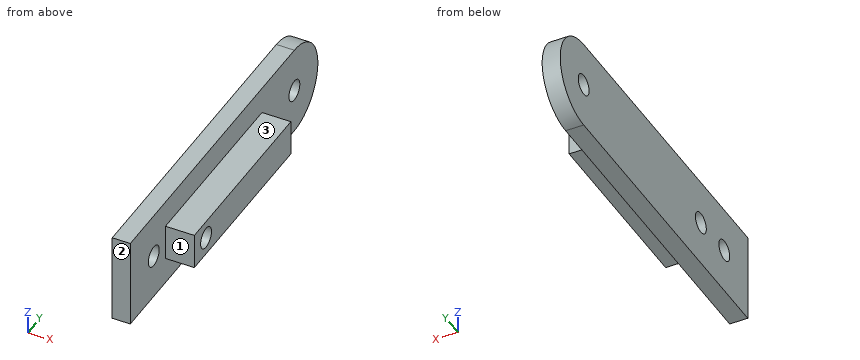
```python
from build123d import *

# Parameters (mm, degrees)
BOSS_EXTRUDE1_DEPTH     = 2.54
SKETCH2_W               = 5.08
SKETCH2_H               = 26.152706233
BOSS_EXTRUDE2_DEPTH     = 4.064
CUT_EXTRUDE1_DEPTH      = 46.384334478
CUT_EXTRUDE1_DEPTH_BACK = 46.384334478
SKETCH3_R               = 1.4732
F_4_CLEARANCE_HOLE1_D   = 2.9464


with BuildPart() as part:
    # Sketch1 → Boss-Extrude1 (new body)
    with BuildSketch(Plane(origin=(0, 0, 0), x_dir=(0, 0, -1), z_dir=(1, 0, 0))):
        with BuildLine():
            Line((-6.35, 0), (-6.35, -44.45))
            Line((-6.35, -44.45), (6.35, -44.45))
            Line((6.35, -44.45), (6.35, 0))
            ThreePointArc((6.35, 0), (0, 6.35), (-6.35, 0))
        make_face()
    extrude(amount=BOSS_EXTRUDE1_DEPTH)

    # Sketch2 → Boss-Extrude2 (add)
    with BuildSketch(Plane(origin=(2.54, 0, 0), x_dir=(0, 0, -1), z_dir=(1, 0, 0))):
        with Locations((0, -21.848646884)):
            Rectangle(SKETCH2_W, SKETCH2_H)
    extrude(amount=BOSS_EXTRUDE2_DEPTH)

    # Sketch3 → Cut-Extrude1 (cut, two sides: drawn at the far end of the back side and taken through both)
    with BuildSketch(Plane.ZY.offset(-CUT_EXTRUDE1_DEPTH_BACK)):
        Circle(SKETCH3_R)
    extrude(amount=CUT_EXTRUDE1_DEPTH + CUT_EXTRUDE1_DEPTH_BACK, mode=Mode.SUBTRACT)

    # #4 Clearance Hole1 (through all)
    with Locations(Plane.ZY):
        with Locations((0, -31.75), (0, -38.1)):
            Hole(F_4_CLEARANCE_HOLE1_D / 2)


solid = part.part
```
Can you work these out from the model? Positions are in its coordinate system, mm. Face numbers are marked on the shaded views. A direction names the side the tool comes from. Round coordinates to 2 decimals unless told otherwise and drop trailing zeros. Loops run counter-clockwise (first coordinate to the right, second up) from the corner with the lowest first, then second, coordinate; pieces in that order, holes last. Notation, with made-up numbers: M 16,42 L 71,42 A29 cw 71,67 Z; hole C -15.75,-34 d1. An arc over 180 degrees is marked long. Answer as a JSON object with one key per item and string values. Group by question number.
Q1. On a 3-axis mill with a long thin cutter (end or side, diameter ignored), from which of +Z, -Z, +X, -X, +Y, -Y can I reach the whole of each face in a straight line? I mean the marked faces 1, 2 and 3. Say none if no direction works.
Q2. Please list where these lines run through material, in increasing order: L1, parallel to Y at x = 0.75, z = 0; L2, parallel to Y at x = 3, z = 0 (3 decimals); L3, parallel to X at y = 2, z = -5.5.
Q3. Will these pins go through, and if not, where does the flat tip stop? pin 1 (2 mm diameter, centred on x = 4, y = -26, fed in from +Z); pin 2 (2.5 mm diameter, centred on y = -38.1, z = 0, fed in from -X); pin 3 (1 mm diameter, centred on x = 4, z = -2, fed in from -Y) (3 decimals); pin 4 (3 mm diameter, centred on y = -38, z = 4, fed in from +X).
Q4. Imagine slicing it at A-A, the plane x = 1. Please give me the cut outline in (y, z).
Q5. Imagine slicing it at B-B, the plane y = -31.75. Please give me the cut outline in (x, z), then the cut area to 3 significant figures.
Q6. Imagine slicing it at D-D, the plane y = -24.5. Please give me the cut outline in (x, z), then the cut area to 3 significant figures.
Q7. Imagine slicing it at C-C, the plane z = 0. Please give me the cut outline in (x, y) (3 decimals).
Findings:
{
 "1": {"face 1": "+Z, -Z, +X, -Y", "face 2": "+Z, -Z, +X, -X, -Y", "face 3": "+Z, +X, +Y, -Y"},
 "2": {"L1": "y = -44.45 to -39.57, -36.63 to -33.22, -30.28 to -1.47, 1.47 to 6.35", "L2": "y = -34.925 to -33.223, -30.277 to -8.772", "L3": "x = 0 to 2.54"},
 "3": {"pin 1": "stops at z = 2.54", "pin 2": "passes through", "pin 3": "stops at y = -34.925", "pin 4": "stops at x = 2.54"},
 "4": {"outline": "M -44.45,-6.35 L 0,-6.35 A6.35 ccw 0,6.35 L -44.45,6.35 Z; hole C -38.1,0 d2.95; hole C -31.75,0 d2.95; hole C 0,0 d2.95"},
 "5": {"outline": "M 0,-6.35 L 2.54,-6.35 L 2.54,-2.54 L 6.6,-2.54 L 6.6,-1.47 L 0,-1.47 Z; M 0,1.47 L 6.6,1.47 L 6.6,2.54 L 2.54,2.54 L 2.54,6.35 L 0,6.35 Z", "area": "33.4 mm2"},
 "6": {"outline": "M 0,-6.35 L 2.54,-6.35 L 2.54,-2.54 L 6.6,-2.54 L 6.6,2.54 L 2.54,2.54 L 2.54,6.35 L 0,6.35 Z", "area": "52.9 mm2"},
 "7": {"outline": "M 0,-44.45 L 2.54,-44.45 L 2.54,-39.573 L 0,-39.573 Z; M 0,-36.627 L 2.54,-36.627 L 2.54,-34.925 L 6.604,-34.925 L 6.604,-33.223 L 0,-33.223 Z; M 0,-30.277 L 6.604,-30.277 L 6.604,-8.772 L 2.54,-8.772 L 2.54,-1.473 L 0,-1.473 Z; M 0,1.473 L 2.54,1.473 L 2.54,6.35 L 0,6.35 Z"}
}
